The model under review builds one solid part; all positions refer to its coordinate system, in mm. Face numbers are marked on the shaded views. Coordinates: 2 decimals unless noted, no trailing zeros. Loops run counter-clockwise (first coordinate to the right, second up) from the corner with the lowest first, then second, coordinate; pieces in that order, holes last. Notation, with made-up numbers: M 39,39 L 80,39 A18 ccw 80,59 Z; hole C -37,84 d1. An arc over 180 degrees is marked long. Write item = value, one per line. Start each with the question number.
Q1. Wall thickness on probe 1 along X at (y, z) = (-6.5, 6); probe 2 along X at (y, z) = (1, 3.5); probe 3 along X at (y, z) = (10.5, 5.5): over which ranges is each line inside the solid? List them lowest first.
Q2. Mouldability with a two-part tool opening along X and no side actions: class the marked faces 1, 2, 3 and 4 as released by +X, released by -X, zero draft, split by the parting line, or undercut.
Q3. We need section A-A on z = 1.25. Give the boundary of the cut face in (x, y), and give its area (3 significant figures).
Q4. Clearance check with a flat-ended pin moving along its axis: pin 1 Ø2.5 at (x, z) = (-17.93, 6) entering from -Y. State where the tip first meets the part, or that it passes through.
Q5. We need section B-B on x = -68.5. Give the boundary of the cut face in (y, z), and give its area (3 significant figures).
from build123d import *

# Parameters (mm, degrees)
SKETCH1_W           = 90
SKETCH1_H           = 100
BOSS_EXTRUDE1_DEPTH = 12
CUT_EXTRUDE4_DEPTH  = 3
LPATTERN1_DEPTH     = 7
SKETCH1_6_R         = 4
CUT_EXTRUDE6_DEPTH  = 121.244349775
SKETCH3_R           = 1.5
CUT_EXTRUDE5_DEPTH  = 145.008145785


# Read off the part's stored shape, not the designer's step: LPattern1
with BuildPart() as part:
    # Sketch1 → Boss-Extrude1 (new body)
    with BuildSketch(Plane.XY):
        with Locations((-57.928839751, 10.994734202)):
            Rectangle(SKETCH1_W, SKETCH1_H)
    extrude(amount=BOSS_EXTRUDE1_DEPTH)

    # Sketch1<5> → Cut-Extrude4 (cut)
    with BuildSketch(Plane.XY):
        with BuildLine():
            Line((-44.928839751, -25.562781554), (-44.928839751, 37.591400024))
            Line((-44.928839751, 37.591400024), (-70.928839751, 11.591400024))
            Line((-70.928839751, 11.591400024), (-70.928839751, -28.377423907))
            Line((-70.928839751, -28.377423907), (-70.928839751, -36.005265798))
            Line((-70.928839751, -36.005265798), (-54.128683309, -36.005265798))
            Line((-54.128683309, -36.005265798), (-45.807519408, -27.684101897))
            ThreePointArc((-45.807519408, -27.684101897), (-45.157201154, -26.710831851), (-44.928839751, -25.562781554))
        make_face()
        Polygon((-50.928839751, 23.10611865), (-50.928839751, -21.987520776), (-56.463060705, -21.011688304), (-64.928839751, -24.092979887), (-64.928839751, 9.10611865), align=None, mode=Mode.SUBTRACT)
    extrude(amount=CUT_EXTRUDE4_DEPTH, mode=Mode.SUBTRACT)

    # LPattern1 outline → LPattern1 (cut)
    with BuildSketch(Plane.XY):
        with BuildLine():
            ThreePointArc((-45.807519408, -17.684101897), (-45.157201154, -16.710831851), (-44.928839751, -15.562781554))
            Line((-44.928839751, -15.562781554), (-44.928839751, 47.591400024))
            Line((-44.928839751, 47.591400024), (-70.928839751, 21.591400024))
            Line((-70.928839751, 21.591400024), (-70.928839751, -26.005265798))
            Line((-70.928839751, -26.005265798), (-54.128683309, -26.005265798))
            Line((-54.128683309, -26.005265798), (-45.807519408, -17.684101897))
        make_face()
        Polygon((-64.928839751, 19.10611865), (-50.928839751, 33.10611865), (-50.928839751, -11.987520776), (-56.463060705, -11.011688304), (-64.928839751, -14.092979887), align=None, mode=Mode.SUBTRACT)
    extrude(amount=LPATTERN1_DEPTH, mode=Mode.SUBTRACT)

    # Sketch1<6> → Cut-Extrude6 (cut, through all)
    with BuildSketch(Plane.XY):
        with Locations((-82.928839751, 45.994734202)):
            Circle(SKETCH1_6_R)
    extrude(amount=CUT_EXTRUDE6_DEPTH, mode=Mode.SUBTRACT)

    # Sketch3 → Cut-Extrude5 (cut, through all)
    with BuildSketch(Plane(origin=(0, 60.994734202, 0), x_dir=(1, 0, 0), z_dir=(0, 1, 0))):
        with Locations(Location((-17.928839751, -6, 0), (0, 0, 270))):
            Circle(SKETCH3_R)
        with Locations(Location((-97.928839751, -6, 0), (0, 0, 270))):
            Circle(SKETCH3_R)
    extrude(amount=-CUT_EXTRUDE5_DEPTH, mode=Mode.SUBTRACT)


solid = part.part
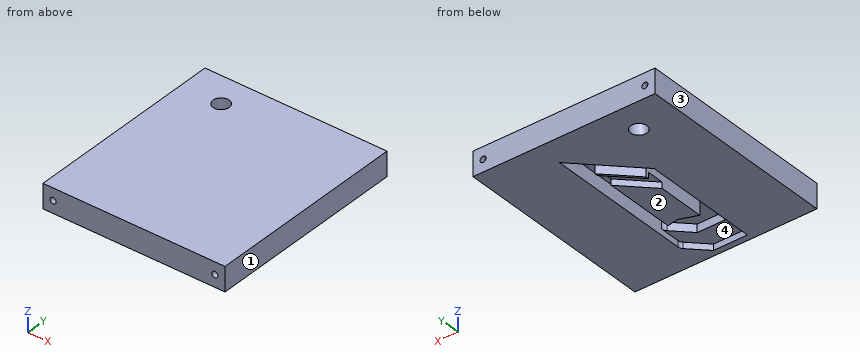
Returned:
q1.probe_1 = -102.93 to -99.43, -96.43 to -70.93, -64.93 to -50.93, -44.93 to -19.43, -16.43 to -12.93
q1.probe_2 = -102.93 to -70.93, -64.93 to -50.93, -44.93 to -12.93
q1.probe_3 = -102.93 to -99.34, -96.51 to -70.93, -64.93 to -50.93, -44.93 to -19.34, -16.51 to -12.93
q2.face_1 = released by +X
q2.face_2 = zero draft
q2.face_3 = released by -X
q2.face_4 = undercut
q3.outline = M -102.93,-39.01 L -12.93,-39.01 L -12.93,60.99 L -102.93,60.99 Z; M -64.93,-14.09 L -56.46,-11.01 L -50.93,-11.99 L -50.93,23.11 L -64.93,9.11 Z; M -64.93,17.59 L -50.93,31.59 L -50.93,33.11 L -64.93,19.11 Z; hole C -82.93,45.99 d8; hole M -70.93,-36.01 L -54.13,-36.01 L -45.81,-27.68 A3 ccw -44.93,-25.56 L -44.93,47.59 L -70.93,21.59 Z
q3.area = 7,570 mm^2
q4.pin_1 = through
q5.outline = M -39.01,0 L -36.01,0 L -36.01,3 L -26.01,3 L -26.01,7 L 24.02,7 L 24.02,0 L 60.99,0 L 60.99,12 L -39.01,12 Z
q5.area = 820 mm^2
